The model under review builds one solid part; all positions refer to its coordinate system, in mm. A direction names the side the tool comes from. Round coordinates to 2 decimals unless told otherwise and drop trailing zeros. Loops run counter-clockwise (first coordinate to the right, second up) from the corner with the lowest first, then second, coordinate; pieces in that order, holes last. Notation, with made-up numbers: M 18,56 L 27,56 A24 cw 27,69 Z; hole C 79,65.25 d9. An arc over 180 degrees is marked long. Answer as a JSON object with one key per item and string values. Group by question number.
Item 1: Tool access review of faces 5 (the face through (-9.66, 17.17, -19.97)), 6 (the face through (-10, 26.335, 4)), 7 (the face through (-20, -8, -15)): name each direction out of +Z, -Z, +X, -X, +Y, -Y from which nothing blocks a thin tool from reaching the whole face with its end or side.
Item 2: Consider section B-B (y = 0). Give the boundary of the cut face in (x, z).
Item 3: Consider section A-A (x = -12.5). Give the boundary of the cut face in (y, z), and give its area (3 significant figures).
Item 4: Consider section C-C (z = -21.5). Give the boundary of the cut face in (x, y), and give its area (3 significant figures).
Item 5: Insertion check: P1, Ø8, axis at x = -15.5, y = 0.5, coming from the +Z side; P2, Ø5, axis at x = -9.5, y = 18.5, coming from the -Z side; P3, Ø3, axis at x = -3, z = -3, coming from the -Y side. Each pin has a flat end and moves straight along its axis. Give the tip position at first contact, or say it passes through.
Item 6: The part is to be moulded in two halves that separate along X. For faces 1 (the face through (1.01, -2.44, 0.54)), 2 (the face through (-21.593, 10, -10)), 3 (the face through (2, 10, -10)), 4 (the face through (-19.593, 9, -9)), say which applies: +X half, -X half, draft (parallel to the pull), parting line (faces both ways), or undercut.
Item 7: To check wall thickness, follow line 1 (Y direction, x = 1.25, z = 0); line 2 (X direction, y = 10.5, z = -9); line 3 (Z direction, x = -8.5, y = 17). State the ranges of each line that lie inside material, in increasing order.
```python
from build123d import *

# Parameters (mm, degrees)
BOSS_EXTRUDE1_DEPTH = 2
BOSS_EXTRUDE2_START = 9.79671523
BOSS_EXTRUDE2_DEPTH = 9.79671523
SKETCH4_R           = 2.5
CUT_EXTRUDE5_DEPTH  = 13


with BuildPart() as part:
    # Sketch1 → Boss-Extrude1 (new body)
    with BuildSketch(Plane(origin=(0, 0, 0), x_dir=(0, 0, -1), z_dir=(1, 0, 0))):
        with BuildLine():
            Line((-8, -4.5), (-8, 28.33511482))
            Line((-8, 28.33511482), (0, 28.33511482))
            ThreePointArc((0, 28.33511482), (21.705957253, 18.213460725), (27.904640757, -4.920341052))
            Line((27.904640757, -4.920341052), (27.361613793, -8))
            Line((27.361613793, -8), (-4.335665421, -8))
            ThreePointArc((-4.335665421, -8), (-5.628363986, -5.685201742), (-8, -4.5))
        make_face()
    extrude(amount=BOSS_EXTRUDE1_DEPTH)

    # Sketch6 → Boss-Extrude2 (add)
    with BuildSketch(Plane.ZY.offset(BOSS_EXTRUDE2_START)):
        with BuildLine():
            Line((8, 26.33511482), (0, 26.33511482))
            ThreePointArc((0, 26.33511482), (-20.173868367, 16.927885506), (-25.935025251, -4.573044697))
            Line((-25.935025251, -4.573044697), (-25.33076057, -8))
            Line((-25.33076057, -8), (-27.361613793, -8))
            Line((-27.361613793, -8), (-27.904640757, -4.920341052))
            ThreePointArc((-27.904640757, -4.920341052), (-21.705957253, 18.213460725), (0, 28.33511482))
            Line((0, 28.33511482), (8, 28.33511482))
            Line((8, 28.33511482), (8, 26.33511482))
        make_face()
    extrude(amount=-BOSS_EXTRUDE2_DEPTH)

    # Mirror1: part across plane


with BuildPart() as part_1:
    add(part.part)
    add(part.part.mirror(Plane.ZY.offset(9.79671523)))

    # Sketch4 → Cut-Extrude5 (cut)
    with BuildSketch(Plane(origin=(2, 0, 0), x_dir=(0, 0, -1), z_dir=(1, 0, 0))):
        Circle(SKETCH4_R)
    extrude(amount=-CUT_EXTRUDE5_DEPTH, mode=Mode.SUBTRACT)


solid = part_1.part
```
Geometry results:
{
 "1": {"face 5": "+Z", "face 6": "+Z, -Y", "face 7": "+Z, -Z, +X, -X, -Y"},
 "2": {"outline": "M -21.59,-28.34 L 2,-28.34 L 2,-2.5 L 0,-2.5 L 0,-26.34 L -19.59,-26.34 L -19.59,8 L -21.59,8 Z; M 0,2.5 L 2,2.5 L 2,8 L 0,8 Z"},
 "3": {"outline": "M -8,-27.36 L -4.92,-27.9 A28.34 ccw 28.34,0 L 28.34,8 L 26.34,8 L 26.34,0 A26.34 cw -4.57,-25.94 L -8,-25.33 Z", "area": "118 mm^2"},
 "4": {"outline": "M -21.59,-8 L -19.59,-8 L -19.59,15.21 L 0,15.21 L 0,-8 L 2,-8 L 2,18.46 L -21.59,18.46 Z", "area": "169 mm^2"},
 "5": {"P1": "stops at z = -25.95", "P2": "stops at z = -23.39", "P3": "stops at y = 25.95"},
 "6": {"face 1": "draft", "face 2": "-X half", "face 3": "+X half", "face 4": "undercut"},
 "7": {"line 1": "y = -8 to -2.5, 2.5 to 28.34", "line 2": "x = -21.59 to -19.59, 0 to 2", "line 3": "z = -22.67 to -20.11"}
}
